Verification items for the finished model (mm, model axes). Round coordinates to 2 decimals unless told otherwise and drop trailing zeros. Order: outer loops, then holes, each group sorted by start corner. A loop starts at its lowest first (then second) coordinate and runs counter-clockwise, first axis right, second up. Notation, with made-up numbers: (-32.5, 7.5) -> (-16.5, 7.5) arc R18 ccw to (-16.5, 11.5) -> close; hole circle Ø8 at (50.5, 48.5). An arc over 180 degrees is marked (long way). Return JSON: item names as keys, results as strings. Group by question number.
Item 1: Depth check by flat-ended pin: pin 1 Ø4 at (y, z) = (41, 5.5) entering from +X; pin 2 Ø4.5 at (x, z) = (-8.5, 6) entering from +Y. Enter the tip coordinate at first touch or a pass-through.
Item 2: Sectioned sample at C-C on y = 42. Record the cut outline in (x, z), plus the area to 3 significant figures.
Item 3: Scan lines: probe 1 along Y at (x, z) = (7.5, 2.5); probe 2 along X at (y, z) = (35.5, 5); probe 3 along Y at (x, z) = (1, 4.25). Record each from-to range of solid material in increasing order. Write a range as from..to.
Item 4: Sectioned sample at A-A on z = 2.5. Record the cut outline in (x, y).
Item 5: Draft check along Y on faces 1 (the flat face through (0, 69.8, 4)), 2 (the flat face through (17.5, 33, 4)), 3 (the flat face through (0, 22, 4)), 4 (the flat face through (1.26, 69.19, 4.44)). Enter one of: pulls with the +Y half, pulls with the -Y half, needs draft (parallel to the pull), parting line crosses it, or undercut.
Item 6: Sectioned sample at B-B on x = -9. Record the cut outline in (y, z).
```python
from build123d import *

# Parameters (mm, degrees)
F0_W      = 50
F0_H      = 30
F1_DEPTH  = 25
F3_DEPTH  = 50
F5_R      = 5
F6_T      = -2.5
F7_R      = 10.7930870798
F8_DEPTH  = 25
F10_DEPTH = 9
F11_W     = 42
F11_H     = 73.1670876886
F12_DEPTH = 22.5


with BuildPart() as f1:
    # F0 (on Top) → F1 (new body)
    with BuildSketch(Plane.XY):
        Rectangle(F0_W, F0_H)
    extrude(amount=F1_DEPTH)


with BuildPart() as f3:
    # F2 (on face) → F3 (new body, through all)
    with BuildSketch(Plane.YZ.offset(25)):
        Polygon((-15, 0), (-15, 25), (-33.741876483, 0), align=None)
    extrude(amount=-F3_DEPTH)


with BuildPart() as f1_1:
    add(f1.part)

    # F4: union F3
    add(f3.part)

    # F5
    f5_edges = [f1_1.edges().sort_by_distance(p)[0] for p in [
        (25, -24.370938, 12.5),
        (-25, -24.370938, 12.5),
        (0, -15, 25),
        (25, 0, 25),
        (-25, 0, 25),
    ]]
    fillet(f5_edges, radius=F5_R)

    # F6
    f6_openings = [f1_1.faces().sort_by_distance(p)[0] for p in [
        (0, -9.243814, 0),
    ]]
    offset(amount=F6_T, openings=f6_openings)

    # F7 (on face) → F8 (cut)
    with BuildSketch(Plane(origin=(0, -21.6015379391, 16.1941342359), x_dir=(1, 0, 0), z_dir=(0, -0.8001247794, 0.5998335914))):
        with Locations((0, -5.4950344037)):
            Circle(F7_R)
    extrude(amount=-F8_DEPTH, mode=Mode.SUBTRACT)


with BuildPart() as f10:
    # F9 (on Top) → F10 (new body)
    with BuildSketch(Plane.XY):
        Polygon((-17.5, 68.6), (-17.5, 22), (17.5, 22), (17.5, 44.3), (17.5, 46.4536678502), (17.5, 68.6), (0.5493581668, 68.6), (-1.4506418332, 68.6), align=None)
        Polygon((17.5, 46.4536678502), (17.5, 44.3), (18.7, 43.3), (18.7, 47.3), align=None)
        Polygon((-2, 69.8), (-1.4506418332, 68.6), (0.5493581668, 68.6), (2, 69.8), align=None)
    extrude(amount=F10_DEPTH)


with BuildPart() as f12:
    # F11 (on Top) → F12 (new body, through all)
    with BuildSketch(Plane.XY):
        with Locations((0, 36.5835438443)):
            Rectangle(F11_W, F11_H)
    extrude(amount=F12_DEPTH)


with BuildPart() as f1_2:
    add(f1_1.part)

    # F13: cut F12
    add(f12.part, mode=Mode.SUBTRACT)


with BuildPart() as f14_1:
    # F14: copy of F1
    add(f1_2.part)


solid = f10.part
```
Recorded:
{
 "1": {"pin 1": "x = 17.5", "pin 2": "y = 68.6"},
 "2": {"outline": "(-17.5, 0) -> (17.5, 0) -> (17.5, 9) -> (-17.5, 9) -> close", "area": "315 mm²"},
 "3": {"probe 1": "22..68.6", "probe 2": "-17.5..17.5", "probe 3": "22..68.6, 68.97..69.8"},
 "4": {"outline": "(-17.5, 22) -> (17.5, 22) -> (17.5, 44.3) -> (18.7, 43.3) -> (18.7, 47.3) -> (17.5, 46.45) -> (17.5, 68.6) -> (0.55, 68.6) -> (2, 69.8) -> (-2, 69.8) -> (-1.45, 68.6) -> (-17.5, 68.6) -> close"},
 "5": {"face 1": "pulls with the +Y half", "face 2": "needs draft", "face 3": "pulls with the -Y half", "face 4": "undercut"},
 "6": {"outline": "(22, 0) -> (68.6, 0) -> (68.6, 9) -> (22, 9) -> close"}
}
